Can you work these out from the model? Positions are in its coordinate system, mm. Round coordinates to 2 decimals unless told otherwise and drop trailing zeros. Loops run counter-clockwise (first coordinate to the right, second up) from the corner with the lowest first, then second, coordinate; pieces in that order, holes last. Notation, with made-up numbers: (3.25, 25.5) -> (46.25, 25.5) arc R12 ccw to (46.25, 44.5) -> close; hole circle Ø9 at (-27, -9.5). An arc over 180 degrees is marked (long way). Write each question's results on one line, items separated by ' | '.
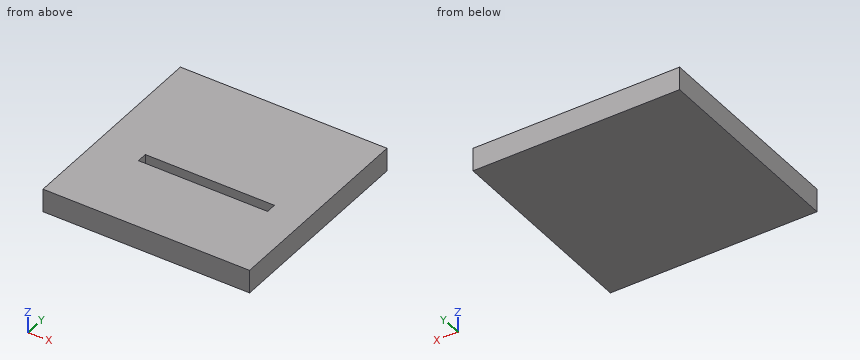
Autodesk Inventor part; units mm, degrees
ref_plane "YZ Plane" through (0, 0, 0) normal (1, 0, 0) x (0, 1, 0)
ref_plane "XZ Plane" through (0, 0, 0) normal (0, 1, 0) x (-1, 0, 0)
ref_plane "XY Plane" through (0, 0, 0) normal (0, 0, 1) x (1, 0, 0)
sketch "Sketch1" plane through (0, 0, 0) normal (0, 0, 1) x (1, 0, 0)
  line L0 (0, 0) -> (400, 0)
  line L1 (400, 0) -> (400, 400)
  line L2 (400, 400) -> (0, 400)
  line L3 (0, 400) -> (0, 0)
  line L4 (135, 150) -> (335, 150)
  line L5 (335, 150) -> (335, 170)
  line L6 (335, 170) -> (135, 170)
  line L7 (135, 170) -> (135, 150)
  dimension "d0" = 400
  dimension "d1" = 400
  dimension "d2" = 200
  dimension "d3" = 20
extrude "Extrusion1" add sketch "Sketch1" along normal blind 40
sketch "Sketch2" plane through (0, 0, 0) normal (0, 0, -1) x (-1, 0, 0)
  line L0 (-400, 0) -> (-400, 400)
  line L1 (0, 400) -> (-400, 400)
  line L2 (-400, 400) -> (-400, 0)
  line L3 (-400, 0) -> (0, 0)
  line L4 (0, 0) -> (0, 400)
extrude "Extrusion2" add sketch "Sketch2" along normal blind 5
sketch "Sketch3" plane through (0, 0, 40) normal (0, 0, 1) x (1, 0, 0)
  line L0 (335, 150) -> (135, 150)
  line L1 (135, 150) -> (85, 150)
  line L2 (85, 150) -> (85, 170)
  line L3 (85, 170) -> (135, 170)
  line L4 (135, 170) -> (135, 150)
  point P0 (0, 0)
  dimension "d8" = 50
  dimension "d9" = 20
extrude "Extrusion3" cut sketch "Sketch3" against normal blind 40
properties part number "basebottomds"
1. If we section it at A-A (z = 15): List the corners of the cut face in (x, y) for me, then the cut area to 3 significant figures.
Final values:
outline: (0, 0) -> (400, 0) -> (400, 400) -> (0, 400) -> close; hole (85, 150) -> (335, 150) -> (335, 170) -> (85, 170) -> close | area: 155,000 mm2
2. Please list where this line runs through material, in increasing order: line 1 (Y direction, x = 118, z = 33). Write a range as from..to.
Final values:
line 1: 0..150, 170..400
3. Will this pin go through, and if not, where does the flat tip stop? pin 1 (6 mm diameter, centred on x = 181, y = 158.5, fed in from +Z).
Final values:
pin 1: z = 0
4. If we section it at B-B (x = 92.5): List the corners of the cut face in (y, z) for me, then the cut area to 3 significant figures.
Final values:
outline: (0, -5) -> (400, -5) -> (400, 40) -> (170, 40) -> (170, 0) -> (150, 0) -> (150, 40) -> (0, 40) -> close | area: 17,200 mm2
